from build123d import *

# Parameters (mm, degrees)
EXTRUDE1_DEPTH               = 30
SKETCH2_W                    = 4.1
SKETCH2_H                    = 60
CUT_FOR_WALKER_CHASSIS_DEPTH = 20.1
F_4_2_4_2_DIAMETER_HOLE1_D   = 4.2
M4X0_7_TAPPED_HOLE1_D        = 4
M4X0_7_TAPPED_HOLE1_DEPTH    = 3.3
SKETCH7_R                    = 1.6
CUT_EXTRUDE1_DEPTH           = 20.1


with BuildPart() as part:
    # Sketch1 → Extrude1 (new body, symmetric)
    with BuildSketch(Plane.XY):
        Polygon((0, 0), (0, 19.1), (3.3, 19.1), (3.3, 3.3), (19.1, 3.3), (19.1, 0), align=None)
    extrude(amount=EXTRUDE1_DEPTH, both=True)

    # Sketch2 → Cut for walker chassis (cut, through all)
    with BuildSketch(Plane.XZ):
        with Locations((17.05, 0)):
            Rectangle(SKETCH2_W, SKETCH2_H)
    extrude(amount=-CUT_FOR_WALKER_CHASSIS_DEPTH, mode=Mode.SUBTRACT)

    # Ø4.2 (4.2) Diameter Hole1 (through all)
    with Locations(Plane.ZY):
        with Locations((-19.5, 7.18), (19.5, 7.18)):
            Hole(F_4_2_4_2_DIAMETER_HOLE1_D / 2)

    # M4x0.7 Tapped Hole1
    with Locations(Plane.XZ):
        with Locations((10, 25), (10, -25)):
            Hole(M4X0_7_TAPPED_HOLE1_D / 2, depth=M4X0_7_TAPPED_HOLE1_DEPTH)

    # Sketch7 → Cut-Extrude1 (cut, through all)
    with BuildSketch(Plane.XZ):
        with Locations((7.25, -12)):
            Circle(SKETCH7_R)
        with Locations((7.25, 12)):
            Circle(SKETCH7_R)
    extrude(amount=-CUT_EXTRUDE1_DEPTH, mode=Mode.SUBTRACT)


solid = part.part
Build history of the part. All positions in model axes, mm. A direction names the side the tool comes from. Give positions to 0.01 mm unless a question says otherwise; leave off trailing zeros. Order: outer loops, then holes, each group sorted by start corner. A loop starts at its lowest first (then second) coordinate and runs counter-clockwise, first axis right, second up. Notation, with made-up numbers: M 50,69.25 L 109,69.25 A18 cw 109,104.25 Z; hole C -11.75,-15.5 d9. An arc over 180 degrees is marked long. Put each result on its own line as item: value.
Item 1: Two-plate mould, pull along Y, no slides. Class faces 1 (the flat face through (2, 19.1, 0)), 2 (the cylindrical face through (1.673, 5.317, 18.531)), 3 (the flat face through (15, 2, 0)), 4 (the flat face through (8, 0, 0)): +Y half, -Y half, draft (parallel to the pull), parting line (faces both ways), or undercut.
From the geometry:
face 1: +Y half
face 2: undercut
face 3: draft
face 4: -Y half
Item 2: Slice it at B-B, the plane x = 7.25. Write the cut outline in (y, z).
From the geometry:
outline: M 0,-30 L 3.3,-30 L 3.3,-13.6 L 0,-13.6 Z; M 0,-10.4 L 3.3,-10.4 L 3.3,10.4 L 0,10.4 Z; M 0,13.6 L 3.3,13.6 L 3.3,30 L 0,30 Z
Item 3: Flat gauge pins, fed straight in: pin 1 Ø3 at (x, z) = (10, -25) entering from +Y; pin 2 Ø1 at (y, z) = (10, 23) entering from +X; pin 3 Ø6 at (x, z) = (8.5, -1.5) entering from +Y. Where does each tip first touch, or does it go through?
From the geometry:
pin 1: passes through
pin 2: stops at x = 3.3
pin 3: stops at y = 3.3
Item 4: 3-axis set-ups, long thin cutter, end or side, ignore diameter. For faces 5 (the flat face through (3.3, 11, 0)), 6 (the flat face through (3, 6, -30)): which of +Z, -Z, +X, -X, +Y, -Y reach the whole face in a straight line?
From the geometry:
face 5: +Z, -Z, +X, +Y
face 6: -Z, +X, -X, +Y, -Y
Item 5: Slice it at C-C, the plane z = 2. Write the cut outline in (x, y), plus the area to 3 significant figures.
From the geometry:
outline: M 0,0 L 15,0 L 15,3.3 L 3.3,3.3 L 3.3,19.1 L 0,19.1 Z
area: 102 mm2
Item 6: Slice it at A-A, the plane z = 25. Write the cut outline in (x, y).
From the geometry:
outline: M 0,0 L 8,0 L 8,3.3 L 3.3,3.3 L 3.3,19.1 L 0,19.1 Z; M 12,0 L 15,0 L 15,3.3 L 12,3.3 Z
Item 7: Slice it at D-D, the plane z = -19.5. Write the cut outline in (x, y), plus the area to 3 significant figures.
From the geometry:
outline: M 0,0 L 15,0 L 15,3.3 L 3.3,3.3 L 3.3,5.08 L 0,5.08 Z; M 0,9.28 L 3.3,9.28 L 3.3,19.1 L 0,19.1 Z
area: 87.8 mm2
Item 8: Probe line 1 (Z direction, x = 10, y = 1.7); line 2 (Z direction, x = 7.25, y = 1.1); line 3 (Y direction, x = 6.5, z = 10). List the from-to ranges inside material, lowest first. Write a range as [from, to].
From the geometry:
line 1: z = [-30, -27], [-23, 23], [27, 30]
line 2: z = [-30, -13.6], [-10.4, 10.4], [13.6, 30]
line 3: y = [0, 3.3]
